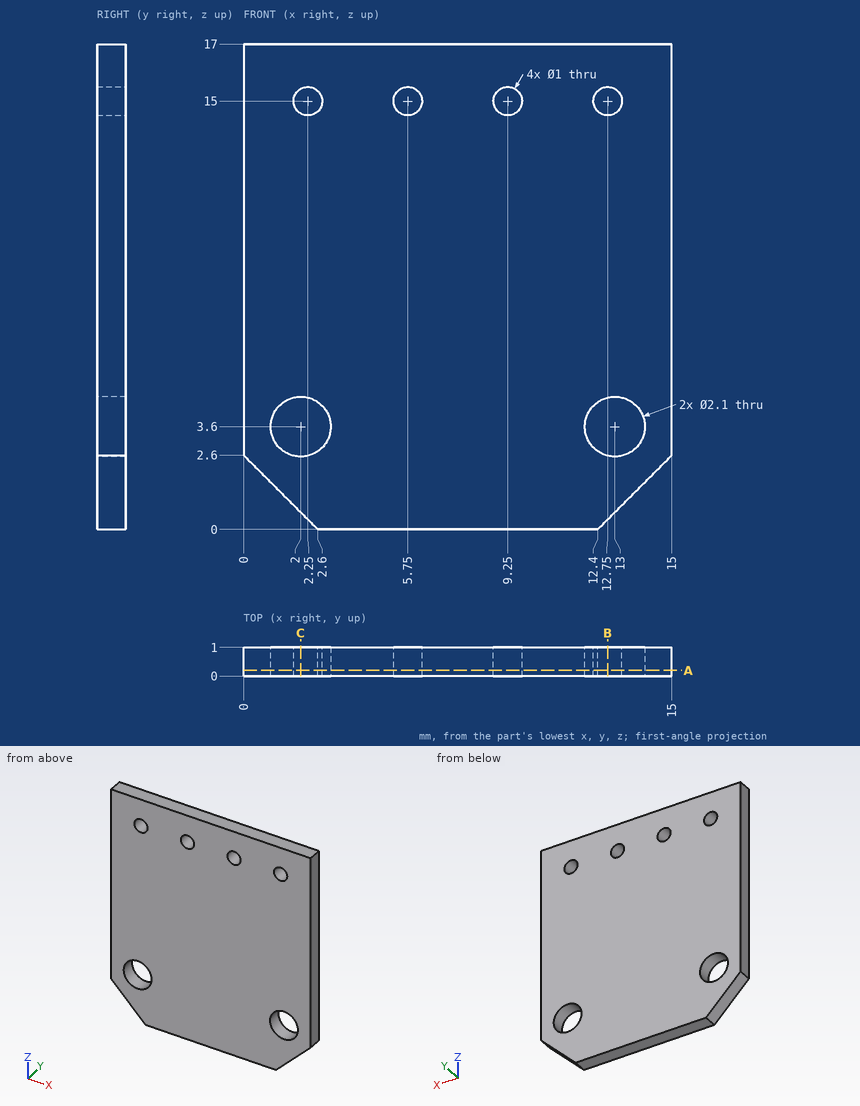
Could you check a few things on this drawing? It's one solid part, dimensions in mm from its lowest x, y, z. Coordinates: 2 decimals unless noted, no trailing zeros. Write each loop counter-clockwise with the first axis right and the second up, starting at its lowest first coordinate (ties: lowest second). Pieces come first, ordered by that corner, then holes. Notation, with made-up numbers: M 53,-32 L 99,-32 A27 ccw 99,3 Z; hole C 42,61.25 d8. An arc over 180 degrees is marked long. Answer as CSV lines item,"result". Start each with the question number.
Q1. I need wall thicknesses on probe 1 along X at (y, z) = (0.6, 15); probe 2 along Z at (x, y) = (13, 0.45); probe 3 along Z at (x, y) = (9.25, 0.55). Which ranges of each line are inside material? Lowest first, please. Write a range as [from, to].
Q2. Suppose I cut it at A-A, the plane y = 0.2. List the corners of the cut face in (x, z) for me, then the cut area to 3 significant figures.
Q3. Suppose I cut it at B-B, the plane x = 12.75. List the corners of the cut face in (y, z) for me, then the cut area to 3 significant figures.
Q4. Suppose I cut it at C-C, the plane x = 2. List the corners of the cut face in (y, z) for me.
Q5. Will this pin go through, and if not, where does the flat tip stop? pin 1 Ø2.5 at (x, z) = (13, 3.6) entering from +Y.
Entries:
1,probe 1,"x = [0, 1.75], [2.75, 5.25], [6.25, 8.75], [9.75, 12.25], [13.25, 15]"
1,probe 2,"z = [0.6, 2.55], [4.65, 14.57], [15.43, 17]"
1,probe 3,"z = [0, 14.5], [15.5, 17]"
2,outline,"M 0,2.6 L 2.6,0 L 12.4,0 L 15,2.6 L 15,17 L 0,17 Z; hole C 2,3.6 d2.1; hole C 2.25,15 d1; hole C 5.75,15 d1; hole C 9.25,15 d1; hole C 13,3.6 d2.1; hole C 12.75,15 d1"
2,area,"238 mm²"
3,outline,"M 0,0.35 L 1,0.35 L 1,2.58 L 0,2.58 Z; M 0,4.62 L 1,4.62 L 1,14.5 L 0,14.5 Z; M 0,15.5 L 1,15.5 L 1,17 L 0,17 Z"
3,area,"13.6 mm²"
4,outline,"M 0,0.6 L 1,0.6 L 1,2.55 L 0,2.55 Z; M 0,4.65 L 1,4.65 L 1,14.57 L 0,14.57 Z; M 0,15.43 L 1,15.43 L 1,17 L 0,17 Z"
5,pin 1,"stops at y = 1"
